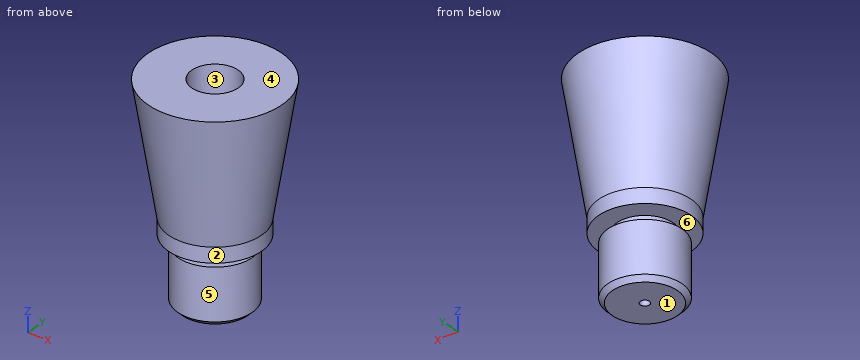
from build123d import *

# Parameters (mm, degrees)
F2_R     = 0.5
F3_DEPTH = 25
F4_R     = 2.5
F4_R_2   = 0.5
F5_DEPTH = 8
F6_SIZE  = 0.5


with BuildPart() as f1:
    # F0 (on Front) → F1 (revolve)
    with BuildSketch(Plane.XZ):
        Polygon((0, 0), (0, 22.5), (-7.2, 22.5), (-5, 8.609747), (-5, 7), (-3, 7), (-3, 6), (-4, 6), (-4, 0), align=None)
    revolve(axis=Axis((0, 0, 11.25), (0, 0, 1)))

    # F2 (on Top) → F3 (cut)
    with BuildSketch(Plane.XY):
        Circle(F2_R)
    extrude(amount=F3_DEPTH, mode=Mode.SUBTRACT)

    # F4 (on face) → F5 (cut)
    with BuildSketch(Plane.XY.offset(22.5)):
        Circle(F4_R)
        Circle(F4_R_2, mode=Mode.SUBTRACT)
    extrude(amount=-F5_DEPTH, mode=Mode.SUBTRACT)

    # F6
    f6_edges = [f1.edges().sort_by_distance(p)[0] for p in [
        (4, 0, 0),
    ]]
    chamfer(f6_edges, length=F6_SIZE)


solid = f1.part
Part model, mm, in its own coordinate system. Face numbers are marked on the shaded views. A direction names the side the tool comes from. Coordinates: 2 decimals unless noted, no trailing zeros. Order: outer loops, then holes, each group sorted by start corner. A loop starts at its lowest first (then second) coordinate and runs counter-clockwise, first axis right, second up.
(1) Pull direction Z, two halves, no side cores. Call the marked faces 4, 5 and 6: pulls with the +Z half, pulls with the -Z half, needs draft (parallel to the pull), parting line crosses it, or undercut.
Check sheet entries:
face 4: pulls with the +Z half
face 5: needs draft
face 6: undercut
(2) Slice it at D-D, the plane z = 16.5. Write the cut outline in (x, y).
Check sheet entries:
outline: circle Ø12.5 at (0, 0); hole circle Ø5 at (0, 0)
(3) Probe L1, parallel to Y at x = 0, z = 8.25; L2, parallel to Y at x = 0, z = 6.5; L3, parallel to Z at x = -3.75, y = 0.75. List the from-to ranges inside material, lowest first.
Check sheet entries:
L1: y = -5 to -0.5, 0.5 to 5
L2: y = -3 to -0.5, 0.5 to 3
L3: z = 0.32 to 6, 7 to 22.5
(4) Pin check, flat tips, straight feed: pin 1 Ø4 at (x, y) = (0, 0) entering from +Z; pin 2 Ø3 at (x, z) = (-1, 13) entering from +Y; pin 3 Ø4 at (x, z) = (-4.5, 18) entering from +Y. Stop position of each tip, or through.
Check sheet entries:
pin 1: stops at z = 14.5
pin 2: stops at y = 5.9
pin 3: stops at y = 6.05
(5) Slice it at A-A, the plane x = 0. Write the cut outline in (y, z).
Check sheet entries:
outline: (-7.2, 22.5) - (-5, 8.61) - (-5, 7) - (-3, 7) - (-3, 6) - (-4, 6) - (-4, 0.5) - (-3.5, 0) - (-0.5, 0) - (-0.5, 14.5) - (-2.5, 14.5) - (-2.5, 22.5) - close; (0.5, 0) - (3.5, 0) - (4, 0.5) - (4, 6) - (3, 6) - (3, 7) - (5, 7) - (5, 8.61) - (7.2, 22.5) - (2.5, 22.5) - (2.5, 14.5) - (0.5, 14.5) - close
(6) Tool access for the marked faces 1, 2 and 3: list every direction of +Z, -Z, +X, -X, +Y, -Y with a clear straight run to the whole face (end or side of a thin tool).
Check sheet entries:
face 1: -Z, +X, -X, +Y, -Y
face 2: -Z
face 3: +Z
(7) Slice it at C-C, the plane z = 8. Write the cut outline in (x, y), and give its area (3 significant figures).
Check sheet entries:
outline: circle Ø10 at (0, 0); hole circle Ø1 at (0, 0)
area: 77.8 mm2
